Part model, mm, in its own coordinate system. Coordinates: 2 decimals unless noted, no trailing zeros. Loops run counter-clockwise (first coordinate to the right, second up) from the corner with the lowest first, then second, coordinate; pieces in that order, holes last. Notation, with made-up numbers: (50, 10.25) - (82, 10.25) arc R17 cw to (82, 34.25) - close; hole circle Ø7 at (-26.5, -15.75). An arc over 180 degrees is marked (long way). Use a Markdown table: item, result. Add a question column.
1) Drop flat-ended pins along their axis: P1, Ø1.5, axis at x = -4.5, y = 2, coming from the -Z side; P2, Ø1.5, axis at x = -6, y = -1.5, coming from the -Z side. Give the stop position or say it passes through.
2) Pull direction X, two halves, no side cores. Call faces 1 (the face through (-19.05, 0, 0)), 2 (the face through (13.97, -2.52, -0.33)), 3 (the face through (19.05, 0, 0)), 4 (the face through (15.13, -3.1, 0.69)): +X half, -X half, draft (parallel to the pull), parting line (faces both ways), or undercut.
3) Probe probe 1 along X at (y, z) = (-2, 2); probe 2 along X at (y, z) = (2, -1.75); probe 3 along Y at (x, z) = (15, -1.75). List the from-to ranges inside material, lowest first. Write a range as [from, to].
4) Band-saw the part on A-A (x = 0.5). Give the cut face in (y, z) (3 decimals), plus the area to 3 significant figures.
from build123d import *

# Parameters (mm, degrees)
EXTRUDE1_DEPTH      = 19.05
EXTRUDE1_DEPTH_BACK = 19.05
SKETCH2_R           = 3.175
CHAMFER1_SIZE       = 0.635
FILLET1_R           = 0.0254


with BuildPart() as part:
    # Sketch2 → Extrude1 (new, two sides: drawn at the far end of the back side and taken through both)
    with BuildSketch(Plane(origin=(0, 0, 0), x_dir=(0, 0, -1), z_dir=(1, 0, 0)).offset(-EXTRUDE1_DEPTH_BACK)):
        Circle(SKETCH2_R)
    extrude(amount=EXTRUDE1_DEPTH + EXTRUDE1_DEPTH_BACK)

    # Chamfer1
    chamfer1_edges = [part.edges().sort_by_distance(p)[0] for p in [
        (-19.05, 0, 3.175),
        (19.05, 0, 3.175),
    ]]
    chamfer(chamfer1_edges, length=CHAMFER1_SIZE)

    # Sketch3 → Cut-Revolve1 (revolve, cut)
    with BuildSketch(Plane.XY, mode=Mode.PRIVATE) as cut_revolve1_sk:
        with BuildLine():
            Line((14.593409285, 2.54), (14.593409285, 3.175))
            Line((14.593409285, 3.175), (11.118656598, 3.175))
            add(Edge.make_bspline(
                [(11.118656598, 3.175), (11.987913735, 3.175), (12.0733688, 2.54), (13.323409285, 2.54)],
                knots=[0, 0, 0, 0, 1, 1, 1, 1], degree=3))
            Line((13.323409285, 2.54), (14.593409285, 2.54))
        make_face()
        with BuildLine():
            Line((19.05, 3.175), (15.662226672, 3.175))
            add(Edge.make_bspline(
                [(15.662226672, 3.175), (16.642763194, 3.175), (18.613991134, 1.631073428), (19.044096366, 1.382495278), (19.05, 1.348727309), (19.05, 1.243390408)],
                knots=[0, 0, 0, 0, 0.565725481, 0.665725481, 1, 1, 1, 1], degree=3))
            Line((19.05, 1.243390408), (19.05, 3.175))
        make_face()
    revolve(cut_revolve1_sk.sketch.rotate(Axis((-19.05, 0, 0), (1, 0, 0)), 90), axis=Axis((-19.05, 0, 0), (1, 0, 0)), mode=Mode.SUBTRACT)

    # Fillet1
    fillet1_edges = [part.edges().sort_by_distance(p)[0] for p in [
        (14.593409285, 0, 3.175),
    ]]
    fillet(fillet1_edges, radius=FILLET1_R)


solid = part.part
Answer block:
| question | item | result |
|---|---|---|
| 1 | P1 | z = -2.92 |
| 1 | P2 | z = -3.09 |
| 2 | face 1 | -X half |
| 2 | face 2 | undercut |
| 2 | face 3 | +X half |
| 2 | face 4 | draft |
| 3 | probe 1 | [-18.76, 12.13], [14.59, 16.79] |
| 3 | probe 2 | [-18.93, 12.52], [14.59, 17.11] |
| 3 | probe 3 | [-2.65, 2.65] |
| 4 | outline | circle Ø6.35 at (0, 0) |
| 4 | area | 31.7 mm2 |
